from build123d import *

# Parameters (mm, degrees)
F1_DEPTH = 17
F4_DEPTH = 14
F3_R     = 3.2
F5_DEPTH = 10
F7_R     = 3.2
F8_DEPTH = 10
F9_R     = 1


with BuildPart() as f1:
    # F0 (on Top) → F1 (new body)
    with BuildSketch(Plane.XY):
        Polygon((0, 80), (0, 0), (50, 0), (100, 0), (100, 80), (50, 80), align=None)
    extrude(amount=F1_DEPTH)

    # F3 (on offset) → F4 (cut)
    with BuildSketch(Plane.XY.offset(17)):
        Polygon((50, 80), (12, 80), (12, 12), (50, 12), (88, 12), (88, 80), align=None)
    extrude(amount=-F4_DEPTH, mode=Mode.SUBTRACT)

    # F3 (on offset) → F5 (cut)
    with BuildSketch(Plane.XY.offset(17)):
        with Locations((6, 6)):
            Circle(F3_R)
        with Locations((94, 6)):
            Circle(F3_R)
    extrude(amount=-F5_DEPTH, mode=Mode.SUBTRACT)

    # F7 (on offset) → F8 (cut)
    with BuildSketch(Plane.XZ.offset(-80)):
        with Locations((94, 6)):
            Circle(F7_R)
        with Locations((6, 6)):
            Circle(F7_R)
    extrude(amount=F8_DEPTH, mode=Mode.SUBTRACT)

    # F9
    f9_edges = [f1.edges().sort_by_distance(p)[0] for p in [
        (12, 46, 3),
        (88, 46, 3),
        (50, 12, 3),
        (90.8, 6, 17),
        (2.8, 6, 17),
        (90.8, 80, 6),
        (2.8, 80, 6),
        (100, 40, 0),
        (50, 0, 0),
        (0, 40, 0),
        (100, 0, 8.5),
        (0, 0, 8.5),
    ]]
    fillet(f9_edges, radius=F9_R)


solid = f1.part
For this review, take the finished solid that the model builds, in its own axes (mm). A direction names the side the tool comes from. Round coordinates to 2 decimals unless told otherwise and drop trailing zeros. Write each loop counter-clockwise with the first axis right and the second up, starting at its lowest first coordinate (ties: lowest second). Pieces come first, ordered by that corner, then holes. Notation, with made-up numbers: (59.25, 2.5) - (95.25, 2.5) arc R16 cw to (95.25, 23.5) - close; hole circle Ø5 at (62.25, 85). An arc over 180 degrees is marked (long way). Write item = value, one per line. Start each with the question number.
1. For faces 1 (the face through (94, 6, 7)), 2 (the face through (49, 12, 11)), 3 (the face through (5.306, 74.563, 2.876)), 4 (the face through (46, 11, 17)), 5 (the face through (100, 40, 9)), list the 3-axis set-ups (+Z, -Z, +X, -X, +Y, -Y) from which the entire face can be reached by the end or side of a thin tool; tool diameter is ignored.
2. Consider section B-B on y = 6. State the section outline as (x, z) points.
3. Draft analysis for pull direction X (two halves, no side actions). For faces 6 (the face through (0, 41, 9)), 7 (the face through (96.956, 4.774, 11.563)), 8 (the face through (12, 46, 11)), 9 (the face through (49, 41, 0)), state which applies: released by +X, released by -X, zero draft, split by the parting line, or undercut.
4. Consider section C-C on x = 6. State the section outline as (y, z) points, plus the area to 3 significant figures.
5. For pin 1 Ø4 at (x, z) = (37.5, 13) entering from +Y; pin 2 Ø5 at (x, y) = (95.5, 6) entering from +Z; pin 3 Ø4 at (x, y) = (6, 6) entering from +Z; pin 4 Ø5 at (x, z) = (7.5, 5) entering from +Y, all flat-tipped, find the tip position at first contact; note any pin that passes through.
6. Wall thickness on L1, parallel to Z at x = 94, y = 76; L2, parallel to X at y = 45, z = 5.5; L3, parallel to Y at x = 94, z = 12: over which ranges is each line inside the solid? List them lowest first.
7. Consider section D-D on y = 50.5. State the section outline as (x, z) points, plus the area to 3 significant figures.
8. Consider section A-A on z = 14. State the section outline as (x, y) points.
Evaluation:
q1.face_1 = +Z
q1.face_2 = +Z, +Y
q1.face_3 = +Y
q1.face_4 = +Z, +X, -X, +Y, -Y
q1.face_5 = +Z, -Z, +X, +Y, -Y
q2.outline = (0, 1) arc R1 ccw to (1, 0) - (99, 0) arc R1 ccw to (100, 1) - (100, 17) - (98.2, 17) arc R1 ccw to (97.2, 16) - (97.2, 7) - (90.8, 7) - (90.8, 16) arc R1 ccw to (89.8, 17) - (10.2, 17) arc R1 ccw to (9.2, 16) - (9.2, 7) - (2.8, 7) - (2.8, 16) arc R1 ccw to (1.8, 17) - (0, 17) - close
q3.face_6 = released by -X
q3.face_7 = undercut
q3.face_8 = undercut
q3.face_9 = zero draft
q4.outline = (0, 1) arc R1 ccw to (1, 0) - (80, 0) - (80, 1.8) arc R1 ccw to (79, 2.8) - (70, 2.8) - (70, 9.2) - (79, 9.2) arc R1 ccw to (80, 10.2) - (80, 17) - (10.2, 17) arc R1 ccw to (9.2, 16) - (9.2, 7) - (2.8, 7) - (2.8, 16) arc R1 ccw to (1.8, 17) - (0, 17) - close
q4.area = 1,230 mm2
q5.pin_1 = 12
q5.pin_2 = 16.98
q5.pin_3 = 7
q5.pin_4 = 80
q6.L1 = 0 to 2.8, 9.2 to 17
q6.L2 = 0 to 12, 88 to 100
q6.L3 = 0 to 2.8, 9.2 to 80
q7.outline = (0, 1) arc R1 ccw to (1, 0) - (99, 0) arc R1 ccw to (100, 1) - (100, 17) - (88, 17) - (88, 4) arc R1 cw to (87, 3) - (13, 3) arc R1 cw to (12, 4) - (12, 17) - (0, 17) - close
q7.area = 636 mm2
q8.outline = (0, 1) arc R1 ccw to (1, 0) - (99, 0) arc R1 ccw to (100, 1) - (100, 80) - (88, 80) - (88, 12) - (12, 12) - (12, 80) - (0, 80) - close; hole circle Ø6.4 at (6, 6); hole circle Ø6.4 at (94, 6)
